Geometry: final body of the model. Coordinates: model frame, mm. A direction names the side the tool comes from. Give positions to 0.01 mm unless a question says otherwise; leave off trailing zeros. Order: outer loops, then holes, each group sorted by start corner. A loop starts at its lowest first (then second) coordinate and runs counter-clockwise, first axis right, second up. Notation, with made-up numbers: (-24.75, -9.75) -> (-16.75, -9.75) arc R16 ccw to (-16.75, 6.25) -> close; hole circle Ø9 at (86, 84.5). An arc over 180 degrees is marked (long way). Write item = value, one per line.
```python
from build123d import *

# Parameters (mm, degrees)
SKETCH1_W           = 150
SKETCH1_H           = 150
BOSS_EXTRUDE1_DEPTH = 250
SHELL1_T            = -10
SKETCH3_W           = 120
SKETCH3_H           = 220
SKETCH3_W_2         = 110
SKETCH3_H_2         = 210
BOSS_EXTRUDE2_DEPTH = 0.001
SKETCH4_W           = 70
SKETCH4_H           = 10
BOSS_EXTRUDE3_DEPTH = 40
SKETCH5_R           = 5
BOSS_EXTRUDE4_DEPTH = 30
SKETCH6_R           = 5
CUT_EXTRUDE2_DEPTH  = 30
SKETCH7_R           = 5
BOSS_EXTRUDE5_DEPTH = 30
SKETCH8_R           = 5
CUT_EXTRUDE3_DEPTH  = 30
SKETCH9_R           = 5
BOSS_EXTRUDE6_DEPTH = 30
SKETCH10_R          = 0.875
CUT_EXTRUDE4_DEPTH  = 145


with BuildPart() as part:
    # Sketch1 → Boss-Extrude1 (new body)
    with BuildSketch(Plane.XY):
        with Locations((75, 75)):
            Rectangle(SKETCH1_W, SKETCH1_H)
    extrude(amount=BOSS_EXTRUDE1_DEPTH)

    # Shell1
    shell1_openings = [part.faces().sort_by_distance(p)[0] for p in [
        (75, 150, 125),
    ]]
    offset(amount=SHELL1_T, openings=shell1_openings, kind=Kind.INTERSECTION)

    # Sketch3 → Boss-Extrude2 (add)
    with BuildSketch(Plane(origin=(0, 0, 0), x_dir=(1, 0, 0), z_dir=(0, 1, 0))):
        with Locations((75, -125)):
            Rectangle(SKETCH3_W, SKETCH3_H)
        with Locations((75, -125)):
            Rectangle(SKETCH3_W_2, SKETCH3_H_2, mode=Mode.SUBTRACT)
    extrude(amount=BOSS_EXTRUDE2_DEPTH)

    # Sketch4 → Boss-Extrude3 (add)
    with BuildSketch(Plane(origin=(0, 0, 0), x_dir=(1, 0, 0), z_dir=(0, 1, 0))):
        with Locations((75, -235)):
            Rectangle(SKETCH4_W, SKETCH4_H)
        with Locations((75, -15)):
            Rectangle(SKETCH4_W, SKETCH4_H)
    extrude(amount=BOSS_EXTRUDE3_DEPTH)

    # Sketch5 → Boss-Extrude4 (add)
    with BuildSketch(Plane.ZY):
        with Locations((0, 150)):
            Circle(SKETCH5_R)
    extrude(amount=-BOSS_EXTRUDE4_DEPTH)

    # Sketch6 → Cut-Extrude2 (cut)
    with BuildSketch(Plane(origin=(30, 0, 0), x_dir=(0, 0, -1), z_dir=(1, 0, 0))):
        with Locations((0, 150)):
            Circle(SKETCH6_R)
    extrude(amount=CUT_EXTRUDE2_DEPTH, mode=Mode.SUBTRACT)

    # Sketch7 → Boss-Extrude5 (add)
    with BuildSketch(Plane.ZY.offset(-60)):
        with Locations((0, 150)):
            Circle(SKETCH7_R)
    extrude(amount=-BOSS_EXTRUDE5_DEPTH)

    # Sketch8 → Cut-Extrude3 (cut)
    with BuildSketch(Plane(origin=(90, 0, 0), x_dir=(0, 0, -1), z_dir=(1, 0, 0))):
        with Locations((0, 150)):
            Circle(SKETCH8_R)
    extrude(amount=CUT_EXTRUDE3_DEPTH, mode=Mode.SUBTRACT)

    # Sketch9 → Boss-Extrude6 (add)
    with BuildSketch(Plane.ZY.offset(-120)):
        with Locations((0, 150)):
            Circle(SKETCH9_R)
    extrude(amount=-BOSS_EXTRUDE6_DEPTH)

    # Sketch10 → Cut-Extrude4 (cut)
    with BuildSketch(Plane.ZY):
        with Locations((0, 150)):
            Circle(SKETCH10_R)
    extrude(amount=-CUT_EXTRUDE4_DEPTH, mode=Mode.SUBTRACT)


solid = part.part
```
1) Reachability of faces 4 (the face through (8, 150, 118)), 5 (the face through (90, 150.07, 1.04)), 6 (the face through (75, 25, 230)) from +Z, -Z, +X, -X, +Y, -Y: full face, straight path, thin tool, end or side. Return the list, or none.
Check sheet entries:
face_4 = +Z, +X, -X, +Y
face_5 = -Z, +Y
face_6 = +Y
2) First-contact query: P1, Ø10, axis at x = 87.5, y = 28.5, coming from the -Z side; P2, Ø10, axis at x = 98, z = 165.5, coming from the +Y side; P3, Ø8, axis at x = 65, z = 13, coming from the +Y side. Flat tips, straight axial feed; report the tip coordinate or a pass-through.
Check sheet entries:
P1 = 0
P2 = 10
P3 = 150
3) Section query A-A (y = 105). Output: boundary loops of the cut face in (x, z), plus the area to 3 significant figures.
Check sheet entries:
outline = (0, 0) -> (150, 0) -> (150, 250) -> (0, 250) -> close; hole (10, 10) -> (140, 10) -> (140, 240) -> (10, 240) -> close
area = 7,600 mm²
4) Section query D-D (x = 136). Output: boundary loops of the cut face in (y, z) (3 decimals).
Check sheet entries:
outline = (0, 0) -> (145, 0) arc R5 ccw (long way) to (150, 5) -> (150, 10) -> (10, 10) -> (10, 240) -> (150, 240) -> (150, 250) -> (0, 250) -> close; hole circle Ø1.75 at (150, 0)
5) Section query C-C (z = 205). Output: boundary loops of the cut face in (x, y).
Check sheet entries:
outline = (0, 0) -> (150, 0) -> (150, 150) -> (140, 150) -> (140, 10) -> (10, 10) -> (10, 150) -> (0, 150) -> close
6) Section query B-B (x = 66.5). Output: boundary loops of the cut face in (y, z) (3 decimals).
Check sheet entries:
outline = (0, 0) -> (145, 0) arc R5 ccw (long way) to (150, 5) -> (150, 10) -> (40, 10) -> (40, 20) -> (10, 20) -> (10, 230) -> (40, 230) -> (40, 240) -> (150, 240) -> (150, 250) -> (0, 250) -> close; hole circle Ø1.75 at (150, 0)
7) Mould query, pull axis X, two halves, no side actions, for faces 1 (the face through (150, 79, 121)), 2 (the face through (74, 81, 240)), 3 (the face through (74, 74, 0)). Classes: +X half, -X half, draft (parallel to the pull), parting line (faces both ways), or undercut.
Check sheet entries:
face_1 = +X half
face_2 = undercut
face_3 = draft
8) Line query: line 1 (X direction, y = 96, z = 37); line 2 (Z direction, x = 134, y = 93); line 3 (Z direction, x = 59, y = 34). Output: solid intervals per line, ascending. Write a range as from..to.
Check sheet entries:
line_1 = 0..10, 140..150
line_2 = 0..10, 240..250
line_3 = 0..20, 230..250
